Geometry: final body of the model. Coordinates: model frame, mm. Give positions to 0.01 mm unless a question says otherwise; leave off trailing zeros. Write each loop counter-clockwise with the first axis right and the second up, starting at its lowest first coordinate (ties: lowest second). Pieces come first, ordered by that corner, then holes. Notation, with made-up numbers: M 8.25,39.25 L 54.25,39.25 A28 ccw 54.25,76.25 Z; hole C -30,-7.75 d2. An arc over 180 degrees is marked long. Use a Markdown table: item, result. Add a question column.
1) Draft query along X for faces 1 (the cylindrical face through (147.15, 9.86, -71.99)), 2 (the flat face through (-2, 20, -1)), 3 (the cylindrical face through (111.7, 9.86, 51.84)). Return one class per face: +X half, -X half, draft (parallel to the pull), parting line (faces both ways), or undercut.
2) Section B-B on y = 7.75. Return the cut outline in (x, z), then the cut area to 3 significant figures.
3) Section C-C on z = -50. Return the cut outline in (x, y), then the cut area to 3 significant figures.
4) Line query: line 1 (X direction, y = 9.25, z = -50). Output: solid intervals per line, ascending.
5) Section A-A on x = 120. Return the cut outline in (y, z).
```python
from build123d import *

# Parameters (mm, degrees)
SALIENTE_EXTRUIR2_DEPTH             = 20
DI_METRO_DE_TALADRO_17_0_17_1_D     = 17
DI_METRO_DE_TALADRO_17_0_17_1_DEPTH = 20


with BuildPart() as part:
    # Croquis1 → Saliente-Extruir2 (new body)
    with BuildSketch(Plane(origin=(0, 0, 0), x_dir=(1, 0, 0), z_dir=(0, 1, 0))):
        with BuildLine():
            Line((140, 75), (-140, 75))
            ThreePointArc((-140, 75), (-147.071067812, 72.071067812), (-150, 65))
            Line((-150, 65), (-150, -65))
            ThreePointArc((-150, -65), (-147.071067812, -72.071067812), (-140, -75))
            Line((-140, -75), (140, -75))
            ThreePointArc((140, -75), (147.071067812, -72.071067812), (150, -65))
            Line((150, -65), (150, 65))
            ThreePointArc((150, 65), (147.071067812, 72.071067812), (140, 75))
        make_face()
    extrude(amount=SALIENTE_EXTRUIR2_DEPTH)

    # Diámetro de taladro Ø17.0 (17)1
    with Locations(Plane(origin=(-120, 20, -50), x_dir=(0, 0, 1), z_dir=(0, 1, 0))):
        with Locations((0, 0), (100, 0), (100, 240), (0, 240)):
            Hole(DI_METRO_DE_TALADRO_17_0_17_1_D / 2, depth=DI_METRO_DE_TALADRO_17_0_17_1_DEPTH)


solid = part.part
```
Found:
| question | item | result |
|---|---|---|
| 1 | face 1 | +X half |
| 1 | face 2 | draft |
| 1 | face 3 | undercut |
| 2 | outline | M -150,-65 A10 ccw -140,-75 L 140,-75 A10 ccw 150,-65 L 150,65 A10 ccw 140,75 L -140,75 A10 ccw -150,65 Z; hole C -120,-50 d17; hole C -120,50 d17; hole C 120,-50 d17; hole C 120,50 d17 |
| 2 | area | 44,000 mm² |
| 3 | outline | M -150,0 L -128.5,0 L -128.5,20 L -150,20 Z; M -111.5,0 L 111.5,0 L 111.5,20 L -111.5,20 Z; M 128.5,0 L 150,0 L 150,20 L 128.5,20 Z |
| 3 | area | 5,320 mm² |
| 4 | line 1 | -150 to -128.5, -111.5 to 111.5, 128.5 to 150 |
| 5 | outline | M 0,-75 L 20,-75 L 20,-58.5 L 0,-58.5 Z; M 0,-41.5 L 20,-41.5 L 20,41.5 L 0,41.5 Z; M 0,58.5 L 20,58.5 L 20,75 L 0,75 Z |
